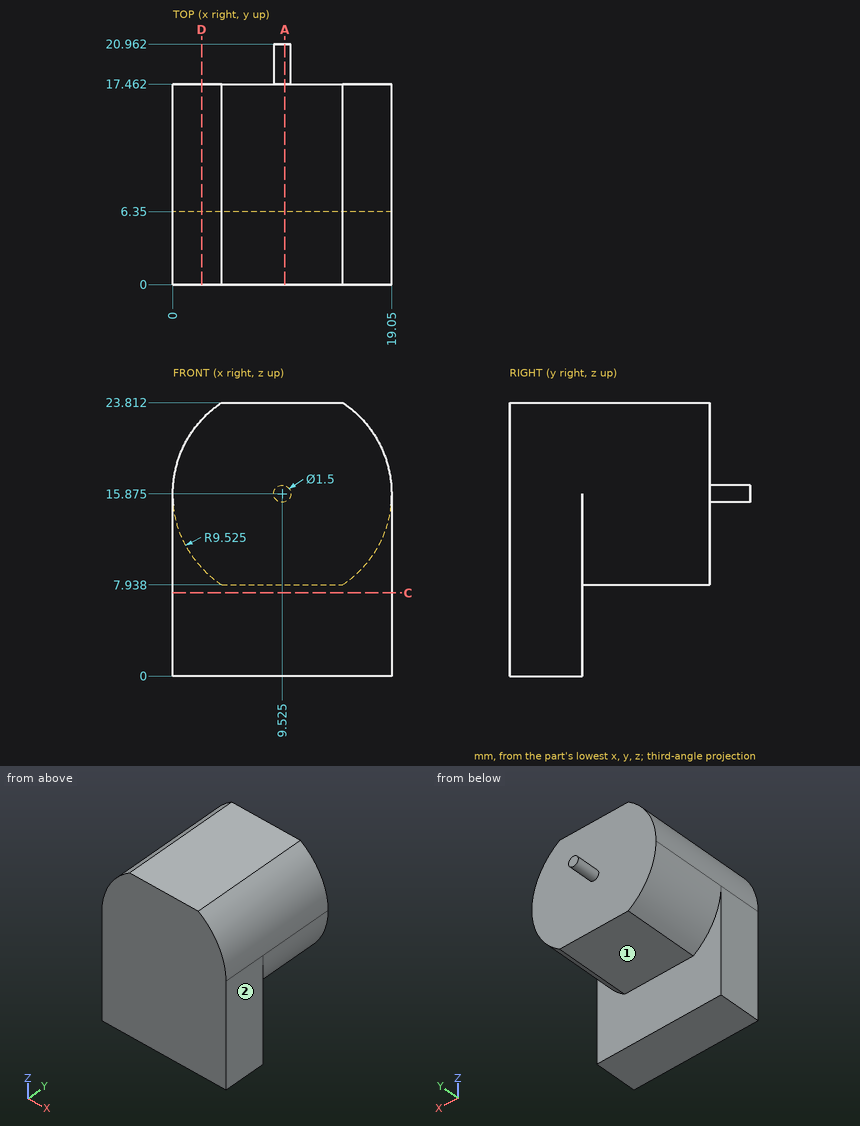
Could you check a few things on this drawing? It's one solid part, dimensions in mm from its lowest x, y, z. A direction names the side the tool comes from. Coordinates: 2 decimals unless noted, no trailing zeros. Order: outer loops, then holes, each group sorted by start corner. A loop starts at its lowest first (then second) coordinate and runs counter-clockwise, first axis right, second up. Notation, with made-up numbers: M -36,17 L 16,17 A14 cw 16,29 Z; hole C -18.75,-35.5 d8. An arc over 180 degrees is marked long. Use a Markdown table: item, result. Add a question column.
Q1. I want a section at D-D on x = 2.5. List the corners of the cut face in (y, z) for me.
Q2. I want a section at C-C on z = 7.25. List the corners of the cut face in (x, y) for me.
Q3. I want a section at A-A on x = 9.75. List the corners of the cut face in (y, z) for me.
Q4. If I drill on L1, parallel to Y at x = 13, z = 1.75; L2, parallel to Y at x = 10.25, z = 18.5; L3, parallel to Z at x = 14.5, y = 16, over which ranges is the centre line in solid material (lowest first)?
Q5. I'm going to push flat-ended pins straight in: pin 1 (8 mm diameter, centred on x = 7, z = 11, fed in from +Y); pin 2 (3 mm diameter, centred on y = 12, z = 6.5, fed in from -X) (1 decimal). Where does each tip first touch, or does it pass through?
Q6. Which directions (+Z, -Z, +X, -X, +Y, -Y) give clear straight access to the entire face, cutting with the end or side of a thin tool? Please do the marked faces 1 and 2.
Checked values:
| question | item | result |
|---|---|---|
| 1 | outline | M 0,0 L 6.35,0 L 6.35,9.44 L 17.46,9.44 L 17.46,22.31 L 0,22.31 Z |
| 2 | outline | M 0,0 L 19.05,0 L 19.05,6.35 L 0,6.35 Z |
| 3 | outline | M 0,0 L 6.35,0 L 6.35,7.94 L 17.46,7.94 L 17.46,15.16 L 20.96,15.16 L 20.96,16.59 L 17.46,16.59 L 17.46,23.81 L 0,23.81 Z |
| 4 | L1 | 0 to 6.35 |
| 4 | L2 | 0 to 17.46 |
| 4 | L3 | 7.94 to 23.81 |
| 5 | pin 1 | y = 17.46 |
| 5 | pin 2 | x = 4.2 |
| 6 | face 1 | -Z, +X, -X, +Y |
| 6 | face 2 | +Z, -Z, +X, +Y, -Y |
